Could you check a few things on this model? Use its own coordinates, in mm. A direction names the side the tool comes from. Coordinates: 2 decimals unless noted, no trailing zeros. Order: outer loops, then holes, each group sorted by start corner. A loop starts at its lowest first (then second) coordinate and runs counter-clockwise, first axis right, second up. Notation, with made-up numbers: (-8, 69) -> (14, 69) arc R14 cw to (14, 90) -> close; hole circle Ø3 at (45, 46.5). An arc over 180 degrees is marked (long way). Put each result on its own line as item: value. Start each with the question number.
Q1. We'd pull the mould along Y, two halves only. Please class faces 6 (the face through (8, -58.557, 5)), 7 (the face through (10.528, -55.466, 6.985)), 8 (the face through (-12.5, -54, 3)): +Y half, -Y half, draft (parallel to the pull), parting line (faces both ways), or undercut.
Q2. Will these pins go through, and if not, where does the flat tip stop? pin 1 (10 mm diameter, centred on x = 28, y = -21.5, fed in from +Z); pin 2 (5 mm diameter, centred on y = -53.5, z = 4.5, fed in from -X); pin 3 (4 mm diameter, centred on x = -12.5, z = 5, fed in from +Y); pin 4 (5 mm diameter, centred on y = -53, z = 4, fed in from +X).
Q3. Please list where these lines run through material, in increasing order: line 1 along X through (y, z) = (-46.5, 2.75); line 2 along X through (y, z) = (0, 2.75); line 3 along Y through (x, z) = (0, 4).
Q4. For faces 1 (the face through (10, -41, 10)), 2 (the face through (-8.21, -49.36, 5.85)), 3 (the face through (-4.5, -48, 5)), 4 (the face through (1.9, 47.21, 4.93)), 5 (the face through (10.53, -48.66, 3.01)), which set-ups out of +Z, -Z, +X, -X, +Y, -Y let a thin tool reach every point of the face, with its end or its side?
Q5. If we section it at B-B (y = 15): Please give me the cut outline in (x, z), and give its area (3 significant figures).
Q6. If we section it at C-C (x = 0): Please give me the cut outline in (y, z).
Q7. If we section it at A-A (y = 0): Please give me the cut outline in (x, z).
Q8. If we section it at D-D (z = 6.25): Count the separate pieces of the cut face and the enclosed holes in it, and give its area (3 significant figures).
from build123d import *

# Parameters (mm, degrees)
F0_R      = 47.25
F0_R_2    = 41.8
F1_DEPTH  = 10
F2_W      = 4.5
F2_H      = 12.6647017896
F3_DEPTH  = 25
F4_W      = 8
F4_H      = 17
F5_DEPTH  = 10
F7_DEPTH  = 4
F8_R      = 2.55
F9_DEPTH  = 25
F10_SIZE2 = 6
F10_SIZE  = 0.7367073654


# Not quite as in the source:
# - a fillet or chamfer that OpenCascade refuses, or shapes differently, is made with other operations: its cross-section is extruded or revolved along the edge and cut away or added


with BuildPart() as f1:
    # F0 (on Top) → F1 (new body)
    with BuildSketch(Plane.XY):
        Circle(F0_R)
        Circle(F0_R_2, mode=Mode.SUBTRACT)
    extrude(amount=F1_DEPTH)

    # F2 (on Top) → F3 (cut)
    with BuildSketch(Plane.XY):
        with Locations((-2.25, -45.0298693031)):
            Rectangle(F2_W, F2_H)
        with Locations((2.25, -45.0298693031)):
            Rectangle(F2_W, F2_H)
    extrude(amount=F3_DEPTH, mode=Mode.SUBTRACT)

    # F4 (on Top) → F5 (join)
    with BuildSketch(Plane.XY):
        with Locations((8.5, -50.0570691941)):
            Rectangle(F4_W, F4_H)
        with Locations((-8.5, -50.0570691941)):
            Rectangle(F4_W, F4_H)
    extrude(amount=F5_DEPTH)

    # F6 (on face) → F7 (cut)
    with BuildSketch(Plane.YZ.offset(12.5)):
        Polygon((-49.7724240202, 1.0679314721), (-47.5118511184, 5.0166414077), (-49.8012477839, 8.9487099356), (-54.3512173512, 8.9320685279), (-56.6117902531, 4.9833585923), (-54.3223935876, 1.0512900644), align=None)
    extrude(amount=-F7_DEPTH, mode=Mode.SUBTRACT)

    # F8 (on face) → F9 (cut)
    with BuildSketch(Plane.YZ.offset(8.5)):
        with Locations((-52.0618206857, 5)):
            Circle(F8_R)
    extrude(amount=-F9_DEPTH, mode=Mode.SUBTRACT)

    # F10
    f10_edges = [f1.edges().sort_by_distance(p)[0] for p in [
        (-4.5, -54.611821, 5),
    ]]
    f10_side = f1.faces().sort_by_distance((-4.5, -50.057069, 0.197231))[0]
    chamfer(f10_edges, length=F10_SIZE, length2=F10_SIZE2, reference=f10_side)

    # F11: chamfer of 6 x 0.6306254116 on 1 edges, made by hand

    # F11_s1 → F11_t2 (revolve, cut)
    with BuildSketch(Plane.XY.offset(5)):
        Polygon((4.5, -48.8811952741), (10.5, -49.5118206857), (4.5, -49.5118206857), align=None)
    revolve(axis=Axis((4.5, -52.0618206857, 5), (1, 0, 0)), mode=Mode.SUBTRACT)


solid = f1.part
The answers:
1. face 6: -Y half
1. face 7: undercut
1. face 8: draft
2. pin 1: through
2. pin 2: x = -12.5
2. pin 3: y = 46.07
2. pin 4: x = 8.5
3. line 1: -12.5 to -4.5, 4.5 to 12.5
3. line 2: -47.25 to -41.8, 41.8 to 47.25
3. line 3: 41.8 to 47.25
4. face 1: +Z, +X, -X, +Y, -Y
4. face 2: none
4. face 3: +Z, -Z, -Y
4. face 4: +Z, -Z
4. face 5: +X
5. outline: (-44.81, 0) -> (-39.02, 0) -> (-39.02, 10) -> (-44.81, 10) -> close; (39.02, 0) -> (44.81, 0) -> (44.81, 10) -> (39.02, 10) -> close
5. area: 116 mm^2
6. outline: (41.8, 0) -> (47.25, 0) -> (47.25, 10) -> (41.8, 10) -> close
7. outline: (-47.25, 0) -> (-41.8, 0) -> (-41.8, 10) -> (-47.25, 10) -> close; (41.8, 0) -> (47.25, 0) -> (47.25, 10) -> (41.8, 10) -> close
8. separate pieces: 3
8. enclosed holes: 0
8. area: 1,580 mm^2
